Here's how the part is built. I have some questions about the finished solid (model axes, mm). Round coordinates to 2 decimals unless told otherwise and drop trailing zeros. Loops run counter-clockwise (first coordinate to the right, second up) from the corner with the lowest first, then second, coordinate; pieces in that order, holes last. Notation, with made-up numbers: (71.5, -19.5) - (99.5, -19.5) arc R29 cw to (99.5, 18.5) - close; hole circle Ø10 at (12.25, 61). An arc over 180 degrees is marked (long way). Answer as a JSON object with one key per item and string values. Group by question number.
1) I want a section at A-A, the plane y = 0. Please give me the cut outline in (x, z), then the cut area to 3 significant figures.
2) I want a section at B-B, the plane x = -20. Please give me the cut outline in (y, z).
3) I want a section at D-D, the plane x = 1. Please give me the cut outline in (y, z).
4) I want a section at C-C, the plane z = 12.7. Please give me the cut outline in (x, y) (1 decimal), then the cut area to 3 significant figures.
5) If I drill on line 1 along X through (y, z) = (19, 17.75); line 2 along Y through (x, z) = (12.5, 12.7); line 3 along Y through (x, z) = (17.5, 16.5), over which ranges is the centre line in solid material (lowest first)? Write a range as [from, to].
6) Will this pin go through, and if not, where does the flat tip stop? P1, Ø5, axis at x = -18.86, y = 18.86, coming from the -Z side.
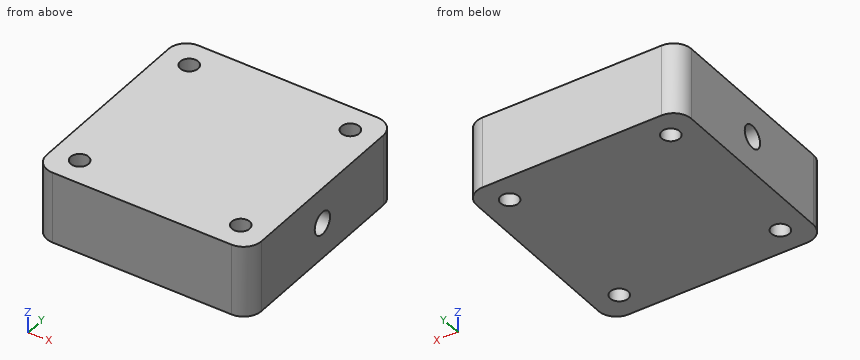
from build123d import *

# Parameters (mm, degrees)
SKETCH1_R           = 3.1877
BOSS_EXTRUDE1_DEPTH = 25.4
SKETCH3_R           = 4
CUT_EXTRUDE1_DEPTH  = 89.9
SCALE1_SCALE        = 0.66


with BuildPart() as part:
    # Sketch1 → Boss-Extrude1 (new body)
    with BuildSketch(Plane.XY):
        with BuildLine():
            Line((-31.75, 38.1), (31.75, 38.1))
            ThreePointArc((31.75, 38.1), (36.240128061, 36.240128061), (38.1, 31.75))
            Line((38.1, 31.75), (38.1, -31.75))
            ThreePointArc((38.1, -31.75), (36.240128061, -36.240128061), (31.75, -38.1))
            Line((31.75, -38.1), (-31.75, -38.1))
            ThreePointArc((-31.75, -38.1), (-36.240128061, -36.240128061), (-38.1, -31.75))
            Line((-38.1, -31.75), (-38.1, 31.75))
            ThreePointArc((-38.1, 31.75), (-36.240128061, 36.240128061), (-31.75, 38.1))
        make_face()
        with Locations((-28.575, 28.575)):
            Circle(SKETCH1_R, mode=Mode.SUBTRACT)
        with Locations((28.575, 28.575)):
            Circle(SKETCH1_R, mode=Mode.SUBTRACT)
        with Locations((28.575, -28.575)):
            Circle(SKETCH1_R, mode=Mode.SUBTRACT)
        with Locations((-28.575, -28.575)):
            Circle(SKETCH1_R, mode=Mode.SUBTRACT)
    extrude(amount=BOSS_EXTRUDE1_DEPTH)

    # Sketch3 → Cut-Extrude1 (cut, through all)
    with BuildSketch(Plane(origin=(38.1, 0, 0), x_dir=(0, 0, -1), z_dir=(1, 0, 0))):
        with Locations((-12.7, 0)):
            Circle(SKETCH3_R)
    extrude(amount=-CUT_EXTRUDE1_DEPTH, mode=Mode.SUBTRACT)


with BuildPart() as part_1:
    # Scale1: scaled about (0, 0, 12.7)
    add(part.part.scale(SCALE1_SCALE).moved(Location((0, 0, 4.318))))


solid = part_1.part
Outcome:
{
 "1": {"outline": "(-25.15, 4.32) - (25.15, 4.32) - (25.15, 10.06) - (-25.15, 10.06) - close; (-25.15, 15.34) - (25.15, 15.34) - (25.15, 21.08) - (-25.15, 21.08) - close", "area": "578 mm^2"},
 "2": {"outline": "(-25.15, 4.32) - (-20.63, 4.32) - (-20.63, 21.08) - (-25.15, 21.08) - close; (-17.09, 4.32) - (17.09, 4.32) - (17.09, 21.08) - (-17.09, 21.08) - close; (20.63, 4.32) - (25.15, 4.32) - (25.15, 21.08) - (20.63, 21.08) - close; hole circle Ø5.28 at (0, 12.7)"},
 "3": {"outline": "(-25.15, 4.32) - (25.15, 4.32) - (25.15, 21.08) - (-25.15, 21.08) - close; hole circle Ø5.28 at (0, 12.7)"},
 "4": {"outline": "(-25.1, -21) arc R4.2 ccw to (-21, -25.1) - (21, -25.1) arc R4.2 ccw to (25.1, -21) - (25.1, -2.6) - (-25.1, -2.6) - close; (-25.1, 2.6) - (25.1, 2.6) - (25.1, 21) arc R4.2 ccw to (21, 25.1) - (-21, 25.1) arc R4.2 ccw to (-25.1, 21) - close; hole circle Ø4.2 at (-18.9, -18.9); hole circle Ø4.2 at (-18.9, 18.9); hole circle Ø4.2 at (18.9, -18.9); hole circle Ø4.2 at (18.9, 18.9)", "area": "2,190 mm^2"},
 "5": {"line 1": "[-25.15, -20.96], [-16.76, 16.76], [20.96, 25.15]", "line 2": "[-25.15, -2.64], [2.64, 25.15]", "line 3": "[-25.15, -20.47], [-17.25, 17.25], [20.47, 25.15]"},
 "6": {"P1": "z = 4.32"}
}
